```python
from build123d import *

# Parameters (mm, degrees)
BOSS_EXTRUDE1_DEPTH      = 2
BOSS_EXTRUDE1_DEPTH_BACK = 2
SKETCH1_R                = 5
SKETCH1_R_2              = 2.5
FILLET1_R                = 0.1
SKETCH2_R                = 4.25
SKETCH2_R_2              = 3.5
CUT_EXTRUDE1_DEPTH       = 0.5


with BuildPart() as part:
    # Sketch1 → Boss-Extrude1 (new, two sides: drawn at the far end of the back side and taken through both)
    with BuildSketch(Plane(origin=(0, 0, 0), x_dir=(1, 0, 0), z_dir=(0, 1, 0)).offset(-BOSS_EXTRUDE1_DEPTH_BACK)):
        with Locations(Location((0, 0, 0), (0, 0, 270))):
            Circle(SKETCH1_R)
        with Locations(Location((0, 0, 0), (0, 0, 270))):
            Circle(SKETCH1_R_2, mode=Mode.SUBTRACT)
    extrude(amount=BOSS_EXTRUDE1_DEPTH + BOSS_EXTRUDE1_DEPTH_BACK)

    # Fillet1
    fillet1_edges = [part.edges().sort_by_distance(p)[0] for p in [
        (0, -2, -5),
        (0, -2, -2.5),
        (0, 2, -5),
        (0, 2, -2.5),
    ]]
    fillet(fillet1_edges, radius=FILLET1_R)

    # Sketch2 → Cut-Extrude1 (cut)
    with BuildSketch(Plane(origin=(0, 2, 0), x_dir=(1, 0, 0), z_dir=(0, 1, 0))):
        with Locations(Location((0, 0, 0), (0, 0, 270))):
            Circle(SKETCH2_R)
        with Locations(Location((0, 0, 0), (0, 0, 270))):
            Circle(SKETCH2_R_2, mode=Mode.SUBTRACT)
    cut_extrude1 = extrude(amount=-CUT_EXTRUDE1_DEPTH, mode=Mode.SUBTRACT)

    # Mirror1: Cut-Extrude1 across plane
    add(cut_extrude1.mirror(Plane.ZX), mode=Mode.SUBTRACT)


solid = part.part
```
Can you work these out from the model? Positions are in its coordinate system, mm. A direction names the side the tool comes from. Round coordinates to 2 decimals unless told otherwise and drop trailing zeros. Loops run counter-clockwise (first coordinate to the right, second up) from the corner with the lowest first, then second, coordinate; pieces in that order, holes last. Notation, with made-up numbers: M 65.25,-1.75 L 102.25,-1.75 A3 ccw 102.25,3.25 Z; hole C 16,53 d6. An arc over 180 degrees is marked long. Answer as a JSON object with one key per item and string values. Group by question number.
Q1. Please list where these lines run through material, in increasing order: L1, parallel to X at y = -1.65, z = 0; L2, parallel to X at y = 1.55, z = -1.5; L3, parallel to X at y = -0.8, z = 0.
Q2. We'd pull the mould along Z, two halves only. Please class faces 1 (the cylindrical face through (-4.88, -0.03, -1.08)), 2 (the flat face through (2, 2, -4)), 3 (the cylindrical face through (4.214, 1.754, -0.553)): +Z half, -Z half, draft (parallel to the pull), parting line (faces both ways), or undercut.
Q3. Will these pins go through, and if not, where does the flat tip stop? pin 1 (4 mm diameter, centred on x = 0, z = 0, fed in from -Y); pin 2 (6 mm diameter, centred on x = 0, z = 0, fed in from +Y); pin 3 (1.5 mm diameter, centred on x = 2.5, y = 0.5, fed in from +Z).
Q4. On a 3-axis mill with a long thin cutter (end or side, diameter ignored), from which of +Z, -Z, +X, -X, +Y, -Y can I reach the whole of each face in a straight line? I mean faces 4 (the flat face through (3, 2, 0)), 5 (the cylindrical face through (-3.417, 1.754, -0.759)), 6 (the cylindrical face through (-3.417, -1.754, -0.759)). Say none if no direction works.
Q5. Imagine slicing it at C-C, the plane y = 0.7. Please give me the cut outline in (x, z).
Findings:
{
 "1": {"L1": "x = -5 to -4.25, -3.5 to -2.5, 2.5 to 3.5, 4.25 to 5", "L2": "x = -4.77 to -3.98, -3.16 to -2, 2 to 3.16, 3.98 to 4.77", "L3": "x = -5 to -2.5, 2.5 to 5"},
 "2": {"face 1": "parting line", "face 2": "draft", "face 3": "undercut"},
 "3": {"pin 1": "passes through", "pin 2": "stops at y = 2", "pin 3": "stops at z = 4.68"},
 "4": {"face 4": "+Z, -Z, +X, -X, +Y", "face 5": "+Y", "face 6": "-Y"},
 "5": {"outline": "C 0,0 d10; hole C 0,0 d5"}
}
